from build123d import *

# Parameters (mm, degrees)
EXTRUDE_1_DEPTH = 5


with BuildPart() as part:
    # 草图1 → 凸台-拉伸1 (new body)
    with BuildSketch(Plane.XY):
        with BuildLine():
            ThreePointArc((39.676398778, 63.242940301), (32.116908157, 65.519966744), (40.007886711, 65.771373436))
            Line((40.007886711, 65.771373436), (81.219528006, 73.870794511))
            ThreePointArc((81.219528006, 73.870794511), (84.756936789, 78.623353252), (89.144446225, 74.642167947))
            ThreePointArc((89.144446225, 74.642167947), (88.550754884, 72.545250848), (86.945915565, 71.070794511))
            Line((86.945915565, 71.070794511), (105.861343633, 33.571373436))
            ThreePointArc((105.861343633, 33.571373436), (109.759730072, 33.406308659), (111.662812973, 30))
            ThreePointArc((111.662812973, 30), (106.761070533, 26.102967723), (104.069382688, 31.757059699))
            Line((104.069382688, 31.757059699), (82.109783132, 42.494523437))
            Line((82.109783132, 42.494523437), (89.614398352, 21.050380059))
            ThreePointArc((89.614398352, 21.050380059), (110.127424639, 10.005834432), (127.344312529, 25.70121614))
            Line((127.344312529, 25.70121614), (103.609378398, 85.394704235))
            ThreePointArc((103.609378398, 85.394704235), (96.558072376, 92.705940943), (86.927534136, 95.93515633))
            Line((86.927534136, 95.93515633), (32.120142981, 85.163730465))
            ThreePointArc((32.120142981, 85.163730465), (15.634853586, 62.961714189), (36.178446258, 44.450768961))
            Line((36.178446258, 44.450768961), (60.302024626, 53.157742297))
            Line((60.302024626, 53.157742297), (39.676398778, 63.242940301))
        make_face()
        with BuildLine():
            Line((81.219528006, 73.870794511), (40.007886711, 65.771373436))
            ThreePointArc((40.007886711, 65.771373436), (40.064153798, 65.387509436), (40.082968492, 65))
            ThreePointArc((40.082968492, 65), (39.98000077, 64.098257559), (39.676398778, 63.242940301))
            Line((39.676398778, 63.242940301), (60.302024626, 53.157742297))
            Line((60.302024626, 53.157742297), (66.852758603, 55.522112342))
            ThreePointArc((66.852758603, 55.522112342), (74.542251323, 55.146923882), (79.686411635, 49.419212353))
            Line((79.686411635, 49.419212353), (82.109783132, 42.494523437))
            Line((82.109783132, 42.494523437), (104.069382688, 31.757059699))
            ThreePointArc((104.069382688, 31.757059699), (104.816909062, 32.810841675), (105.861343633, 33.571373436))
            Line((105.861343633, 33.571373436), (86.945915565, 71.070794511))
            ThreePointArc((86.945915565, 71.070794511), (83.387386526, 71.048737661), (81.219528006, 73.870794511))
        make_face()
    extrude(amount=EXTRUDE_1_DEPTH)


solid = part.part
The listing builds one solid part. Answer for the finished solid, in the listing's coordinates (mm). Coordinates: 2 decimals unless noted, no trailing zeros. Write each loop counter-clockwise with the first axis right and the second up, starting at its lowest first coordinate (ties: lowest second). Pieces come first, ordered by that corner, then holes. Notation, with made-up numbers: (77, -21) - (127, -21) arc R26 ccw to (127, -6) - close; hole circle Ø8 at (67, -11). An arc over 180 degrees is marked (long way). Put each result on its own line as item: value.
1. The part is cut by section B-B on x = 110. Give the vertices of the cut face in (y, z), plus the area to 3 significant figures.
Answer sheet:
outline: (9.99, 0) - (26.75, 0) - (26.75, 5) - (9.99, 5) - close; (33.25, 0) - (69.32, 0) - (69.32, 5) - (33.25, 5) - close
area: 264 mm^2
2. Flat-ended cylindrical pins translate along their axes: pin 1 Ø6.5 at (x, y) = (107.66, 30) entering from +Z; pin 2 Ø3 at (x, z) = (67, 1.5) entering from +Y; pin 3 Ø2 at (y, z) = (56, 4) entering from -X; pin 4 Ø2 at (x, z) = (96.5, 4.5) entering from -Y. Find the tip coordinate at first contact, or state that the pin passes through.
Answer sheet:
pin 1: passes through
pin 2: stops at y = 92.31
pin 3: stops at x = 17.15
pin 4: stops at y = 12.61
3. The part is cut by section A-A on z = 2.85. Give the vertices of the cut face in (x, y), plus the area to 3 significant figures.
Answer sheet:
outline: (32.12, 85.16) arc R20.55 ccw to (36.18, 44.45) - (66.85, 55.52) arc R10 cw to (79.69, 49.42) - (89.61, 21.05) arc R20.15 ccw to (127.34, 25.7) - (103.61, 85.39) arc R21.37 ccw to (86.93, 95.94) - close; hole circle Ø8 at (36.08, 65); hole circle Ø8 at (85.14, 74.64); hole circle Ø8 at (107.66, 30)
area: 4,900 mm^2
4. Find the intervals of material crossed by line 1 along X through (y, z) = (30, 3); line 2 along X through (y, z) = (64, 2.25); line 3 along X through (y, z) = (23.5, 3.65), in increasing order. Write a range as from..to.
Answer sheet:
line 1: x = 86.48..103.66, 111.66..125.64
line 2: x = 15.56..32.21, 39.96..112.12
line 3: x = 88.76..126.73
5. The part is cut by section C-C on y = 46. Give the vertices of the cut face in (x, z).
Answer sheet:
outline: (28.25, 0) - (40.47, 0) - (40.47, 5) - (28.25, 5) - close; (80.88, 0) - (119.27, 0) - (119.27, 5) - (80.88, 5) - close
6. The part is cut by section D-D on y = 82. Give the vertices of the cut face in (x, z), plus the area to 3 significant figures.
Answer sheet:
outline: (24.54, 0) - (104.96, 0) - (104.96, 5) - (24.54, 5) - close
area: 402 mm^2
